from build123d import *

# Parameters (mm, degrees)
F1_DEPTH = 40
F2_R     = 17.49999
F3_R     = 2.5
F4_DEPTH = 25
F5_R     = 1
F6_DEPTH = 25


# Not quite as in the source:
# - a fillet or chamfer is up to 0.001 mm smaller than in the source, because OpenCascade refuses the exact size


with BuildPart() as f1:
    # F0 (on Top) → F1 (new body)
    with BuildSketch(Plane.XY):
        Polygon((17.5, 10), (0, 10), (-17.5, 10), (-17.5, -10), (17.5, -10), align=None)
    extrude(amount=F1_DEPTH)

    # F2 (radius 17.5 in the source; OpenCascade refuses exactly that, so slightly less here)
    f2_edges = [f1.edges().sort_by_distance(p)[0] for p in [
        (17.5, 0, 40),
        (-17.5, 0, 40),
    ]]
    fillet(f2_edges, radius=F2_R)

    # F3 (on face) → F4 (cut)
    with BuildSketch(Plane.XZ.offset(10)):
        with Locations((0, 30)):
            Circle(F3_R)
    extrude(amount=-F4_DEPTH, mode=Mode.SUBTRACT)

    # F5 (on face) → F6 (cut)
    with BuildSketch(Plane(origin=(0, 0, 0), x_dir=(1, 0, 0), z_dir=(0, 0, -1))):
        with Locations((10, 0)):
            Circle(F5_R)
        with Locations((-10, 0)):
            Circle(F5_R)
    extrude(amount=-F6_DEPTH, mode=Mode.SUBTRACT)


solid = f1.part
Source: CAD feature listing. Evaluate the final solid. Frame: model axes, mm. A direction names the side the tool comes from. Round coordinates to 2 decimals unless told otherwise and drop trailing zeros. Loops run counter-clockwise (first coordinate to the right, second up) from the corner with the lowest first, then second, coordinate; pieces in that order, holes last. Notation, with made-up numbers: (43.25, 50.5) - (53.25, 50.5) arc R30 cw to (53.25, 73.5) - close; hole circle Ø4 at (-17.5, -28). An arc over 180 degrees is marked (long way). Write item = value, one per line. Start each with the question number.
(1) Section query B-B, the plane z = 30. Output: boundary loops of the cut face in (x, y).
(2) Section query D-D, the plane z = 24.5. Output: boundary loops of the cut face in (x, y).
(3) Pull-direction query (Y, two-part tool) for faces 3 (the face through (0, 0, 0)), 4 (the face through (-10.8, 0.6, 12.3)), 5 (the face through (0, 10, 20)), 6 (the face through (0, -10, 20)); classes: +Y half, -Y half, draft (parallel to the pull), parting line (faces both ways), or undercut.
(4) Pin query (flat end, axial travel): pin 1 (3 mm diameter, centred on x = 6.5, y = 0.5, fed in from +Z); pin 2 (1.2 mm diameter, centred on x = -10, y = 0, fed in from -Z); pin 3 (1.5 mm diameter, centred on x = -7, y = -6.5, fed in from +Z); pin 4 (4.5 mm diameter, centred on x = 0, z = 30, fed in from +Y). Return the tip coordinate at first contact, or that it passes through.
(5) Section query C-C, the plane x = 10. Output: boundary loops of the cut face in (y, z).
(6) Ray query, line 1 along X through (y, z) = (0, 9.75); line 2 along Z through (x, y) = (0, 2); line 3 along X through (y, z) = (-0.75, 4). Return the intervals inside material, ascending. Write a range as from..to.
(7) Set-up query: faces 1 (the face through (-10, 0, 25)), 2 (the face through (-12.51, -0.14, 34.74)). Return all of +Z, -Z, +X, -X, +Y, -Y with unobstructed straight access to the full face (end or side cutting, diameter ignored); none if empty.
Conclusion:
q1.outline = (-15.81, -10) - (-2.5, -10) - (-2.5, 10) - (-15.81, 10) - close; (2.5, -10) - (15.81, -10) - (15.81, 10) - (2.5, 10) - close
q2.outline = (-17.39, -10) - (17.39, -10) - (17.39, 10) - (-17.39, 10) - close; hole circle Ø2 at (-10, 0); hole circle Ø2 at (10, 0)
q3.face_3 = draft
q3.face_4 = undercut
q3.face_5 = +Y half
q3.face_6 = -Y half
q4.pin_1 = 39.27
q4.pin_2 = 25
q4.pin_3 = 38.85
q4.pin_4 = through
q5.outline = (-10, 0) - (-1, 0) - (-1, 25) - (1, 25) - (1, 0) - (10, 0) - (10, 36.86) - (-10, 36.86) - close
q6.line_1 = -17.5..-11, -9..9, 11..17.5
q6.line_2 = 0..27.5, 32.5..40
q6.line_3 = -17.5..-10.66, -9.34..9.34, 10.66..17.5
q7.face_1 = -Z
q7.face_2 = +Z, -X, +Y, -Y
